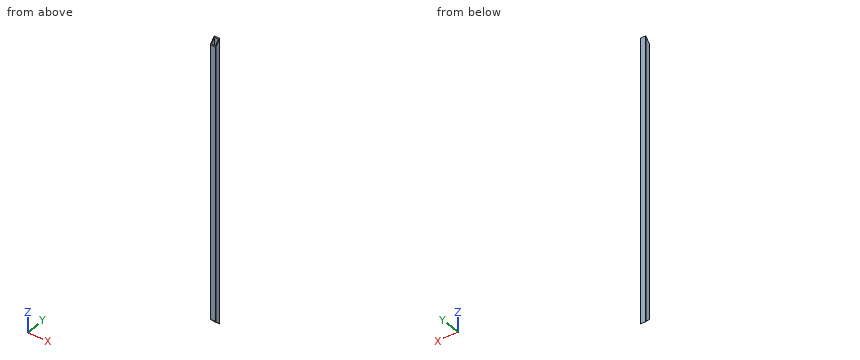
```python
from build123d import *

# Parameters (mm, degrees)
F1_DEPTH = 2565.4
F3_DEPTH = 50.801


with BuildPart() as f1:
    # F0 (on Top) → F1 (new body)
    with BuildSketch(Plane.XY):
        with BuildLine():
            Line((22.225, 25.4), (-22.225, 25.4))
            ThreePointArc((-22.225, 25.4), (-24.470064, 24.470064), (-25.4, 22.225))
            Line((-25.4, 22.225), (-25.4, -22.225))
            ThreePointArc((-25.4, -22.225), (-24.470064, -24.470064), (-22.225, -25.4))
            Line((-22.225, -25.4), (22.225, -25.4))
            ThreePointArc((22.225, -25.4), (24.470064, -24.470064), (25.4, -22.225))
            Line((25.4, -22.225), (25.4, 22.225))
            ThreePointArc((25.4, 22.225), (24.470064, 24.470064), (22.225, 25.4))
        make_face()
        with BuildLine():
            ThreePointArc((-19.05, 17.4625), (-18.585032, 18.585032), (-17.4625, 19.05))
            Line((-17.4625, 19.05), (17.4625, 19.05))
            ThreePointArc((17.4625, 19.05), (18.585032, 18.585032), (19.05, 17.4625))
            Line((19.05, 17.4625), (19.05, -17.4625))
            ThreePointArc((19.05, -17.4625), (18.585032, -18.585032), (17.4625, -19.05))
            Line((17.4625, -19.05), (-17.4625, -19.05))
            ThreePointArc((-17.4625, -19.05), (-18.585032, -18.585032), (-19.05, -17.4625))
            Line((-19.05, -17.4625), (-19.05, 17.4625))
        make_face(mode=Mode.SUBTRACT)
    extrude(amount=F1_DEPTH)

    # F2 (on face) → F3 (cut, through all)
    with BuildSketch(Plane.YZ.offset(25.4)):
        Polygon((-25.4, 2514.6), (25.4, 2565.4), (-25.4, 2565.4), align=None)
        Polygon((-25.4, 0), (25.4, 0), (-25.4, 50.8), align=None)
    extrude(amount=-F3_DEPTH, mode=Mode.SUBTRACT)


solid = f1.part
```
Can you work these out from the model? Positions are in its coordinate system, mm. Coordinates: 2 decimals unless noted, no trailing zeros. Order: outer loops, then holes, each group sorted by start corner. A loop starts at its lowest first (then second) coordinate and runs counter-clockwise, first axis right, second up.
1. If we section it at A-A (y = 8): Please give me the cut outline in (x, z).
2. I need wall thicknesses on line 1 (X direction, y = -8, z = 1655); line 2 (Z direction, x = -17, y = -22.5). Which ranges of each line are inside material? Lowest first, please.
3. If we section it at B-B (x = -2): Please give me the cut outline in (y, z).
4. I'm going to push a flat-ended pin straight in: pin 1 (1 mm diameter, centred on x = -12.5, y = -17, fed in from +Z). Where does the tip first touch, or does it pass through?
Entries:
1. outline: (-25.4, 17.4) - (-19.05, 17.4) - (-19.05, 2548) - (-25.4, 2548) - close; (19.05, 17.4) - (25.4, 17.4) - (25.4, 2548) - (19.05, 2548) - close
2. line 1: x = -25.4 to -19.05, 19.05 to 25.4
2. line 2: z = 47.9 to 2517.5
3. outline: (-25.4, 50.8) - (-19.05, 44.45) - (-19.05, 2520.95) - (-25.4, 2514.6) - close; (19.05, 6.35) - (25.4, 0) - (25.4, 2565.4) - (19.05, 2559.05) - close
4. pin 1: passes through
